from build123d import *

# Parameters (mm, degrees)
F0_W     = 55
F0_H     = 50
F0_R     = 4
F0_W_2   = 12
F1_DEPTH = 25
F2_DEPTH = 43
F3_R     = 1


with BuildPart() as f1:
    # F0 (on Top) → F1 (new body)
    with BuildSketch(Plane.XY):
        Rectangle(F0_W, F0_H)
        with Locations((-18.5, 0)):
            Circle(F0_R, mode=Mode.SUBTRACT)
        with Locations((33.5, 0)):
            Rectangle(F0_W_2, F0_H)
    extrude(amount=F1_DEPTH)

    # F0 (on Top) → F2 (join)
    with BuildSketch(Plane.XY):
        with Locations((33.5, 0)):
            Rectangle(F0_W_2, F0_H)
    extrude(amount=F2_DEPTH)

    # F3
    f3_edges = [f1.edges().sort_by_distance(p)[0] for p in [
        (27.5, 25, 34),
        (33.5, 25, 43),
        (39.5, 25, 21.5),
        (39.5, 0, 43),
        (27.5, 0, 43),
        (33.5, -25, 43),
        (27.5, -25, 34),
        (39.5, -25, 21.5),
    ]]
    fillet(f3_edges, radius=F3_R)


solid = f1.part
Design review of the part built by this model. Coordinates are the model's own, in mm. A direction names the side the tool comes from. Round coordinates to 2 decimals unless told otherwise and drop trailing zeros. Write each loop counter-clockwise with the first axis right and the second up, starting at its lowest first coordinate (ties: lowest second). Pieces come first, ordered by that corner, then holes.
Item 1: Consider section B-B on y = 0. Give the boundary of the cut face in (x, z).
Item 2: Consider section C-C on z = 29.5. Give the boundary of the cut face in (x, y), and give its area (3 significant figures).
Item 3: Consider section D-D on y = -13. Give the boundary of the cut face in (x, z).
Item 4: For faces 4 (the flat face through (6, 0, 0)), 5 (the flat face through (27.5, 0, 33)), list the 3-axis set-ups (+Z, -Z, +X, -X, +Y, -Y) from which the entire face can be reached by the end or side of a thin tool; tool diameter is ignored.
Item 5: For pin 1 Ø25 at (x, y) = (11, -5.5) entering from +Z; pin 2 Ø10 at (y, z) = (-2.5, 35.5) entering from -X, all flat-tipped, find the tip position at first contact; note any pin that passes through.
Item 6: Wall thickness on L1, parallel to Z at x = 7, y = 1.5; L2, parallel to Y at x = -18.5, z = 6.5; L3, parallel to X at y = -4.5, z = 37.5: over which ranges is each line inside the solid? List them lowest first.
Item 7: Draft analysis for pull direction Y (two halves, no side actions). For faces 1 (the cylindrical face through (-21.7, -2.4, 12.3)), 2 (the flat face through (39.5, 0, 21)), 3 (the flat face through (5, -25, 11)), state which applies: released by +Y, released by -Y, zero draft, split by the parting line, or undercut.
Item 8: Consider section A-A on x = -18.5. Give the boundary of the cut face in (y, z).
Check values:
1. outline: (-27.5, 0) - (-22.5, 0) - (-22.5, 25) - (-27.5, 25) - close; (-14.5, 0) - (39.5, 0) - (39.5, 42) arc R1 ccw to (38.5, 43) - (28.5, 43) arc R1 ccw to (27.5, 42) - (27.5, 25) - (-14.5, 25) - close
2. outline: (27.5, -24) arc R1 ccw to (28.5, -25) - (38.5, -25) arc R1 ccw to (39.5, -24) - (39.5, 24) arc R1 ccw to (38.5, 25) - (28.5, 25) arc R1 ccw to (27.5, 24) - close
2. area: 599 mm2
3. outline: (-27.5, 0) - (39.5, 0) - (39.5, 42) arc R1 ccw to (38.5, 43) - (28.5, 43) arc R1 ccw to (27.5, 42) - (27.5, 25) - (-27.5, 25) - close
4. face 4: -Z, +X, -X, +Y, -Y
4. face 5: +Z, -X, +Y, -Y
5. pin 1: stops at z = 25
5. pin 2: stops at x = 27.5
6. L1: z = 0 to 25
6. L2: y = -25 to -4, 4 to 25
6. L3: x = 27.5 to 39.5
7. face 1: undercut
7. face 2: zero draft
7. face 3: released by -Y
8. outline: (-25, 0) - (-4, 0) - (-4, 25) - (-25, 25) - close; (4, 0) - (25, 0) - (25, 25) - (4, 25) - close
